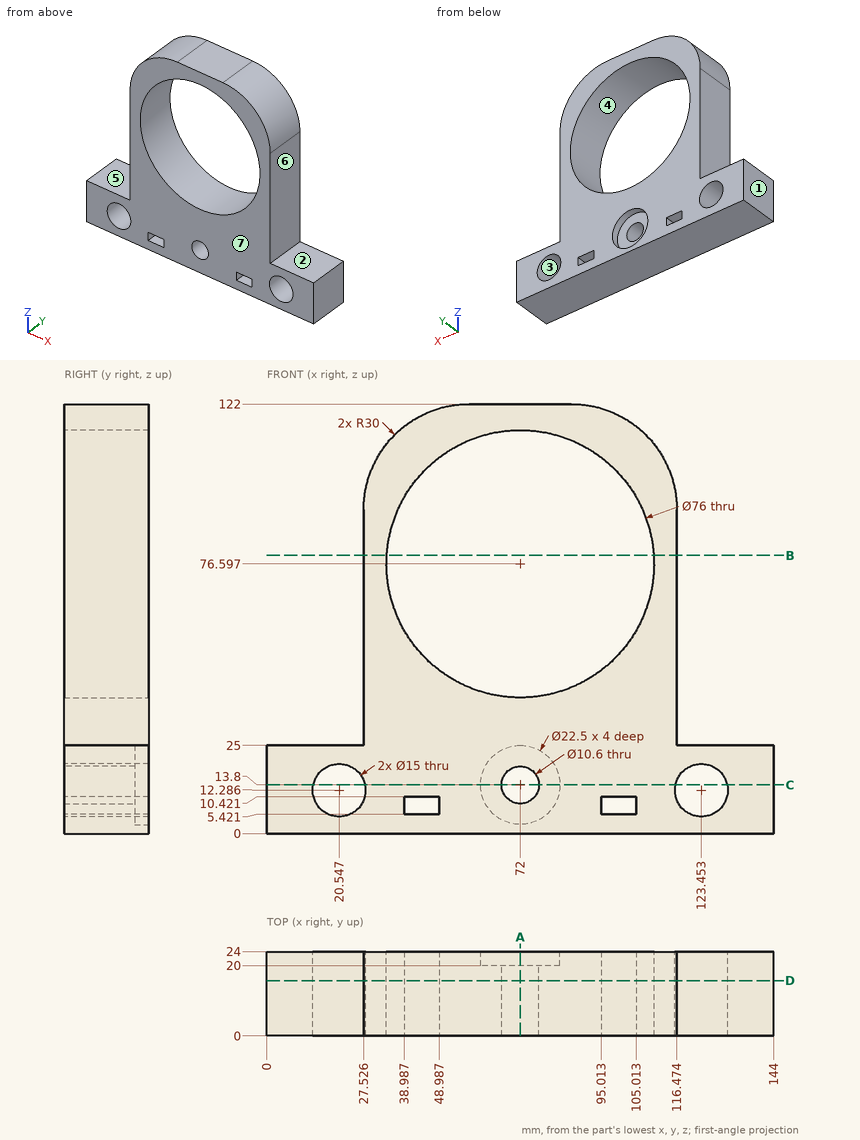
Can you work these out from the drawing? Everything is in mm from the part's minimum corner. A direction names the side the tool comes from. Give positions to 0.01 mm unless a question says otherwise; leave off trailing zeros. Order: outer loops, then holes, each group sorted by start corner. A loop starts at its lowest first (then second) coordinate and runs counter-clockwise, first axis right, second up.
1. Suppose I cut it at C-C (z = 13.8). List the corners of the cut face in (x, y) for me.
2. Suppose I cut it at B-B (z = 79). List the corners of the cut face in (x, y) for me (1 decimal).
3. Will these pins go through, and if not, where does the flat tip stop? P1, Ø4, axis at y = 21.5, z = 57, coming from the -X side; P2, Ø9, axis at x = 123.45, z = 12.29, coming from the +Y side; P3, Ø8, axis at x = 99.5, y = 16, coming from the +Z side; P4, Ø7, axis at x = 14.5, y = 7, coming from the +Z side.
4. Suppose I cut it at D-D (y = 15.75). List the corners of the cut face in (x, z) for me (1 decimal).
5. I need wall thicknesses on L1, parallel to Z at x = 67.5, y = 19 (1 decimal); L2, parallel to Z at x = 124, y = 13.25 (1 decimal); L3, parallel to Z at x = 79, y = 7.5 (1 decimal). Which ranges of each line are inside material? Lowest first, please.
6. For the marked faces 5, 6 and 7, which set-ups out of +Z, -Z, +X, -X, +Y, -Y let a thin tool reach every point of the face, with its end or its side?
7. Suppose I cut it at A-A (x = 72). List the corners of the cut face in (y, z) for me.
8. We'd pull the mould along Z, two halves only. Please class the marked faces 1, 2, 3 and 4: pulls with the +Z half, pulls with the -Z half, needs draft (parallel to the pull), parting line crosses it, or undercut.
Solved:
1. outline: (0, 0) - (13.2, 0) - (13.2, 24) - (0, 24) - close; (27.89, 0) - (66.7, 0) - (66.7, 20) - (60.75, 20) - (60.75, 24) - (27.89, 24) - close; (77.3, 0) - (116.11, 0) - (116.11, 24) - (83.25, 24) - (83.25, 20) - (77.3, 20) - close; (130.8, 0) - (144, 0) - (144, 24) - (130.8, 24) - close
2. outline: (27.5, 0) - (34.1, 0) - (34.1, 24) - (27.5, 24) - close; (109.9, 0) - (116.5, 0) - (116.5, 24) - (109.9, 24) - close
3. P1: stops at x = 27.53
3. P2: passes through
3. P3: stops at z = 120.61
3. P4: stops at z = 25
4. outline: (0, 0) - (144, 0) - (144, 25) - (116.5, 25) - (116.5, 92) arc R30 ccw to (86.5, 122) - (57.5, 122) arc R30 ccw to (27.5, 92) - (27.5, 25) - (0, 25) - close; hole circle Ø15 at (20.5, 12.3); hole circle Ø76 at (72, 76.6); hole (39, 5.4) - (49, 5.4) - (49, 10.4) - (39, 10.4) - close; hole circle Ø10.6 at (72, 13.8); hole (95, 5.4) - (105, 5.4) - (105, 10.4) - (95, 10.4) - close; hole circle Ø15 at (123.5, 12.3)
5. L1: z = 0 to 11, 16.6 to 38.9, 114.3 to 122
5. L2: z = 0 to 4.8, 19.8 to 25
5. L3: z = 0 to 39.2, 113.9 to 122
6. face 5: +Z, -X, +Y, -Y
6. face 6: +Z, +X, +Y, -Y
6. face 7: +Z, -Z, +X, -X, -Y
7. outline: (0, 0) - (24, 0) - (24, 2.55) - (20, 2.55) - (20, 8.5) - (0, 8.5) - close; (0, 19.1) - (20, 19.1) - (20, 25.05) - (24, 25.05) - (24, 38.6) - (0, 38.6) - close; (0, 114.6) - (24, 114.6) - (24, 122) - (0, 122) - close
8. face 1: needs draft
8. face 2: pulls with the +Z half
8. face 3: undercut
8. face 4: undercut
